Check sheet for the drawn part. Datum: minimum x, y, z corner. Units: mm. A direction names the side the tool comes from. Round coordinates to 2 decimals unless told otherwise and drop trailing zeros. Loops run counter-clockwise (first coordinate to the right, second up) from the corner with the lowest first, then second, coordinate; pieces in that order, holes last. Notation, with made-up numbers: (40.25, 69) - (47.25, 69) arc R8 cw to (47.25, 79) - close; hole circle Ø7 at (87.25, 49.25). An arc over 180 degrees is marked (long way). Use CSV: the item, a comma, the result in double quotes.
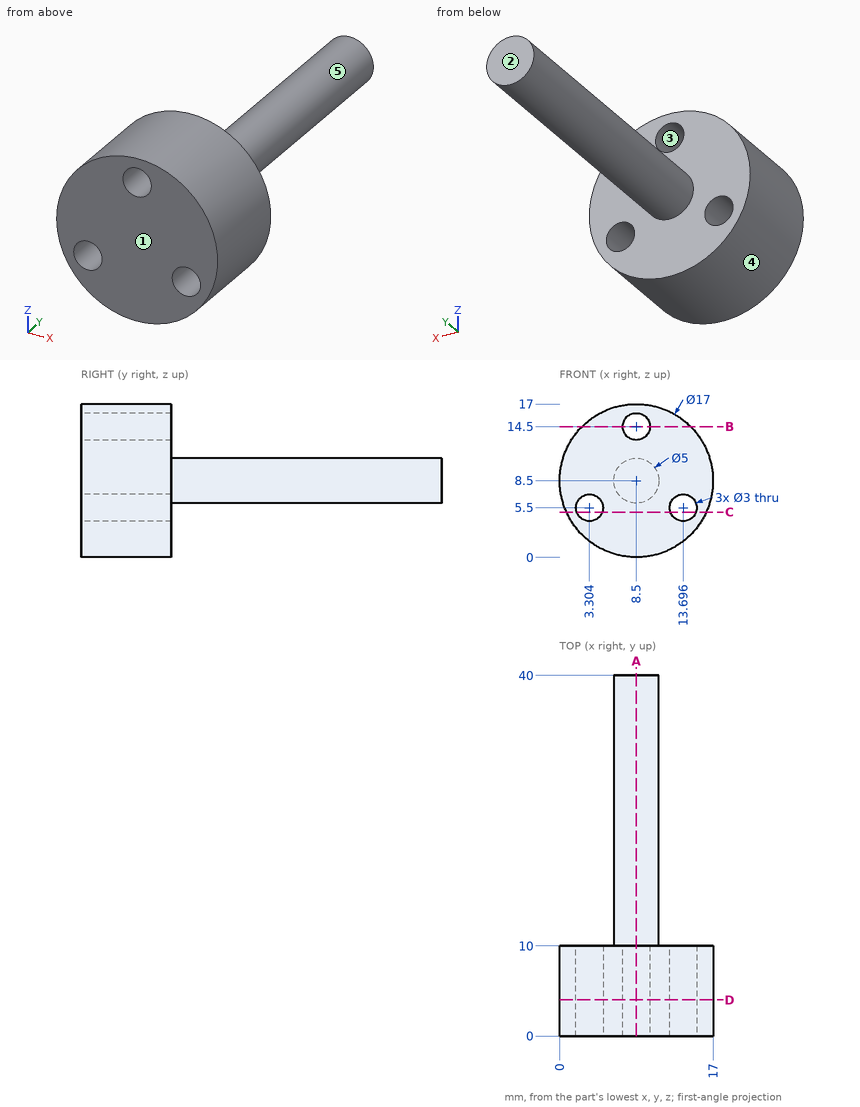
1) Cross-section at A-A, the plane x = 8.5. Record the cut outline in (y, z), then the cut area to 3 significant figures.
Returned:
outline,"(0, 0) - (10, 0) - (10, 6) - (40, 6) - (40, 11) - (10, 11) - (10, 13) - (0, 13) - close; (0, 16) - (10, 16) - (10, 17) - (0, 17) - close"
area,"290 mm²"
2) Mould release check, pull along Y, two halves, no side actions. Record for the marked faces 1, 2 and 3: +Y half, -Y half, draft (parallel to the pull), parting line (faces both ways), or undercut.
Returned:
face 1,"-Y half"
face 2,"+Y half"
face 3,"draft"
3) Access from +Z, -Z, +X, -X, +Y, -Y to the whole of each face (thin tool, end or side, straight path). Record for the marked faces 4 and 5.
Returned:
face 4,"+Y, -Y"
face 5,"+Y"
4) Cross-section at D-D, the plane y = 4. Record the cut outline in (x, z).
Returned:
outline,"circle Ø17 at (8.5, 8.5); hole circle Ø3 at (3.3, 5.5); hole circle Ø3 at (8.5, 14.5); hole circle Ø3 at (13.7, 5.5)"
5) Thickness scan on probe 1 along Z at (x, y) = (8.5, 7); probe 2 along Y at (x, z) = (7.75, 4); probe 3 along Z at (x, y) = (2.5, 4). Record the ranges inside material, lowest first. Write a range as [from, to].
Returned:
probe 1,"z = [0, 13], [16, 17]"
probe 2,"y = [0, 10]"
probe 3,"z = [2.48, 4.23], [6.77, 14.52]"
6) Gauge pin test, flat ends, axial feed: pin 1 Ø2 at (y, z) = (11.5, 10.5) entering from -X; pin 2 Ø8 at (y, z) = (4.5, 2) entering from -X; pin 3 Ø1 at (x, z) = (2, 3) entering from +Y; pin 4 Ø2.5 at (x, z) = (8.5, 14.5) entering from +Y. Record the tip position at first contact, or that the pin passes through.
Returned:
pin 1,"stops at x = 6.21"
pin 2,"stops at x = 0.38"
pin 3,"stops at y = 10"
pin 4,"passes through"
7) Cross-section at C-C, the plane z = 5. Record the cut outline in (x, y).
Returned:
outline,"(0.75, 0) - (1.89, 0) - (1.89, 10) - (0.75, 10) - close; (4.72, 0) - (12.28, 0) - (12.28, 10) - (4.72, 10) - close; (15.11, 0) - (16.25, 0) - (16.25, 10) - (15.11, 10) - close"
8) Cross-section at B-B, the plane z = 14.5. Record the cut outline in (x, y), then the cut area to 3 significant figures.
Returned:
outline,"(2.48, 0) - (7, 0) - (7, 10) - (2.48, 10) - close; (10, 0) - (14.52, 0) - (14.52, 10) - (10, 10) - close"
area,"90.4 mm²"
